Could you check a few things on this model? Use its own coordinates, in mm. A direction names the side the tool comes from. Round coordinates to 2 decimals unless told otherwise and drop trailing zeros. Write each loop counter-clockwise with the first axis right and the second up, starting at its lowest first coordinate (ties: lowest second). Pieces come first, ordered by that corner, then holes. Notation, with made-up numbers: (46.25, 37.25) -> (66.25, 37.25) arc R25 ccw to (66.25, 49.25) -> close; hole circle Ø1 at (66, 15). An arc over 180 degrees is marked (long way). Return JSON: item names as keys, results as strings.
from build123d import *

# Parameters (mm, degrees)
BASE_FLANGE1_DEPTH = 2080


# Sheet-metal steps are written as plain solids
with BuildPart() as part:
    # Sketch1 → Base-Flange1 (new body)
    with BuildSketch(Plane.XY):
        with BuildLine():
            Line((0, 10), (0, 2))
            ThreePointArc((0, 2), (0.585786438, 0.585786438), (2, 0))
            Line((2, 0), (67.5, 0))
            ThreePointArc((67.5, 0), (69.798097039, -0.951902961), (70.75, -3.25))
            Line((70.75, -3.25), (70.75, -94.75))
            ThreePointArc((70.75, -94.75), (69.798097039, -97.048097039), (67.5, -98))
            Line((67.5, -98), (59, -98))
            ThreePointArc((59, -98), (57.585786438, -98.585786438), (57, -100))
            Line((57, -100), (57, -143.5))
            ThreePointArc((57, -143.5), (56.048097039, -145.798097039), (53.75, -146.75))
            Line((53.75, -146.75), (38.25, -146.75))
            ThreePointArc((38.25, -146.75), (35.951902961, -145.798097039), (35, -143.5))
            Line((35, -143.5), (35, -136.75))
            Line((35, -136.75), (36.25, -136.75))
            Line((36.25, -136.75), (36.25, -143.5))
            ThreePointArc((36.25, -143.5), (36.835786438, -144.914213562), (38.25, -145.5))
            Line((38.25, -145.5), (53.75, -145.5))
            ThreePointArc((53.75, -145.5), (55.164213562, -144.914213562), (55.75, -143.5))
            Line((55.75, -143.5), (55.75, -100))
            ThreePointArc((55.75, -100), (56.701902961, -97.701902961), (59, -96.75))
            Line((59, -96.75), (67.5, -96.75))
            ThreePointArc((67.5, -96.75), (68.914213562, -96.164213562), (69.5, -94.75))
            Line((69.5, -94.75), (69.5, -3.25))
            ThreePointArc((69.5, -3.25), (68.914213562, -1.835786438), (67.5, -1.25))
            Line((67.5, -1.25), (2, -1.25))
            ThreePointArc((2, -1.25), (-0.298097039, -0.298097039), (-1.25, 2))
            Line((-1.25, 2), (-1.25, 10))
            Line((-1.25, 10), (0, 10))
        make_face()
    extrude(amount=BASE_FLANGE1_DEPTH)


solid = part.part
1) If I drill on probe 1 along Y at (x, z) = (43, 1014); probe 2 along Y at (x, z) = (64, 1749); probe 3 along X at (y, z) = (-10, 1220.5), over which ranges is the centre line in solid material (lowest first)? Write a range as [from, to].
Return value:
{"probe 1": "[-146.75, -145.5], [-1.25, 0]", "probe 2": "[-98, -96.75], [-1.25, 0]", "probe 3": "[69.5, 70.75]"}
2) Thinking about a two-plate mould opening in Y: for faces 1 (the face through (69.5, -50, 1025)), 2 (the face through (70, -80, 0)), 3 (the face through (34, 0, 1025)), which applies, pulls with the +Y half, pulls with the -Y half, needs draft (parallel to the pull), parting line crosses it, or undercut?
Return value:
{"face 1": "undercut", "face 2": "needs draft", "face 3": "pulls with the +Y half"}
3) I want a section at A-A, the plane z = 743. Please give me the cut outline in (x, y).
Return value:
{"outline": "(-1.25, 2) arc R3.25 ccw to (2, -1.25) -> (67.5, -1.25) arc R2 cw to (69.5, -3.25) -> (69.5, -94.75) arc R2 cw to (67.5, -96.75) -> (59, -96.75) arc R3.25 ccw to (55.75, -100) -> (55.75, -143.5) arc R2 cw to (53.75, -145.5) -> (38.25, -145.5) arc R2 cw to (36.25, -143.5) -> (36.25, -136.75) -> (35, -136.75) -> (35, -143.5) arc R3.25 ccw to (38.25, -146.75) -> (53.75, -146.75) arc R3.25 ccw to (57, -143.5) -> (57, -100) arc R2 cw to (59, -98) -> (67.5, -98) arc R3.25 ccw to (70.75, -94.75) -> (70.75, -3.25) arc R3.25 ccw to (67.5, 0) -> (2, 0) arc R2 cw to (0, 2) -> (0, 10) -> (-1.25, 10) -> close"}
4) For faces 4 (the face through (70, -80, 2080)), 5 (the face through (57, -121, 1025)), 6 (the face through (35, -1.25, 1025)), which set-ups out of +Z, -Z, +X, -X, +Y, -Y let a thin tool reach every point of the face, with its end or its side?
Return value:
{"face 4": "+Z, +X, -X, +Y, -Y", "face 5": "+Z, -Z, +X, -Y", "face 6": "+Z, -Z, -X"}
5) Will these pins go through, and if not, where does the flat tip stop? pin 1 Ø2.5 at (y, z) = (6.5, 1283) entering from +X; pin 2 Ø1 at (x, z) = (17, 734) entering from -Y; pin 3 Ø5.5 at (y, z) = (-139.5, 1344) entering from +X.
Return value:
{"pin 1": "x = 0", "pin 2": "y = -1.25", "pin 3": "x = 57"}
6) I want a section at B-B, the plane x = 20. Please give me the cut outline in (y, z), and give its area (3 significant figures).
Return value:
{"outline": "(-1.25, 0) -> (0, 0) -> (0, 2080) -> (-1.25, 2080) -> close", "area": "2,600 mm²"}
7) I want a section at C-C, the plane y = -50. Please give me the cut outline in (x, z), and give its area (3 significant figures).
Return value:
{"outline": "(69.5, 0) -> (70.75, 0) -> (70.75, 2080) -> (69.5, 2080) -> close", "area": "2,600 mm²"}
